Drawing for the job (mm, zero at the part's lowest x, y, z). A direction names the side the tool comes from. Give positions to 0.01 mm unless a question says otherwise; leave off trailing zeros. Write each loop counter-clockwise with the first axis right and the second up, starting at its lowest first coordinate (ties: lowest second). Pieces come first, ordered by that corner, then holes. Notation, with made-up numbers: M 20,59 L 79,59 A27 cw 79,97 Z; hole C 7.5,-16 d4. An arc over 180 degrees is marked long. Use CSV: the item, a comma, the result in double quotes. Start each with the question number.
1. Band-saw the part on B-B, the plane z = 3.75. List the corners of the cut face in (x, y).
2. Drop flat-ended pins along their axis: pin 1 Ø1.6 at (x, z) = (2.5, 2.5) entering from +Y; pin 2 Ø2 at (x, z) = (12, 2.5) entering from +Y; pin 3 Ø3.5 at (x, z) = (3.75, 11.25) entering from +Y. Give the stop position or say it passes through.
3. Band-saw the part on D-D, the plane y = 7.25. List the corners of the cut face in (x, z), then the cut area to 3 significant figures.
4. Mould opens along Z. For the marked faces 1, 2, 3 and 4 say: pulls with the +Z half, pulls with the -Z half, needs draft (parallel to the pull), parting line crosses it, or undercut.
5. Band-saw the part on C-C, the plane y = 3.5. Count the separate pieces of the cut face and the enclosed holes in it, then the cut area to 3 significant figures.
6. Drill centre lines: line 1 along Z through (x, y) = (3.75, 0.5); line 2 along X through (y, z) = (1.95, 3.75). Where is each one in solid material? Low to high. Write a range as from..to.
7. 3-axis set-ups, long thin cutter, end or side, ignore diameter. For the marked faces 5, 6 and 7: which of +Z, -Z, +X, -X, +Y, -Y reach the whole face in a straight line?
8. Band-saw the part on A-A, the plane x = 3.75. List the corners of the cut face in (y, z).
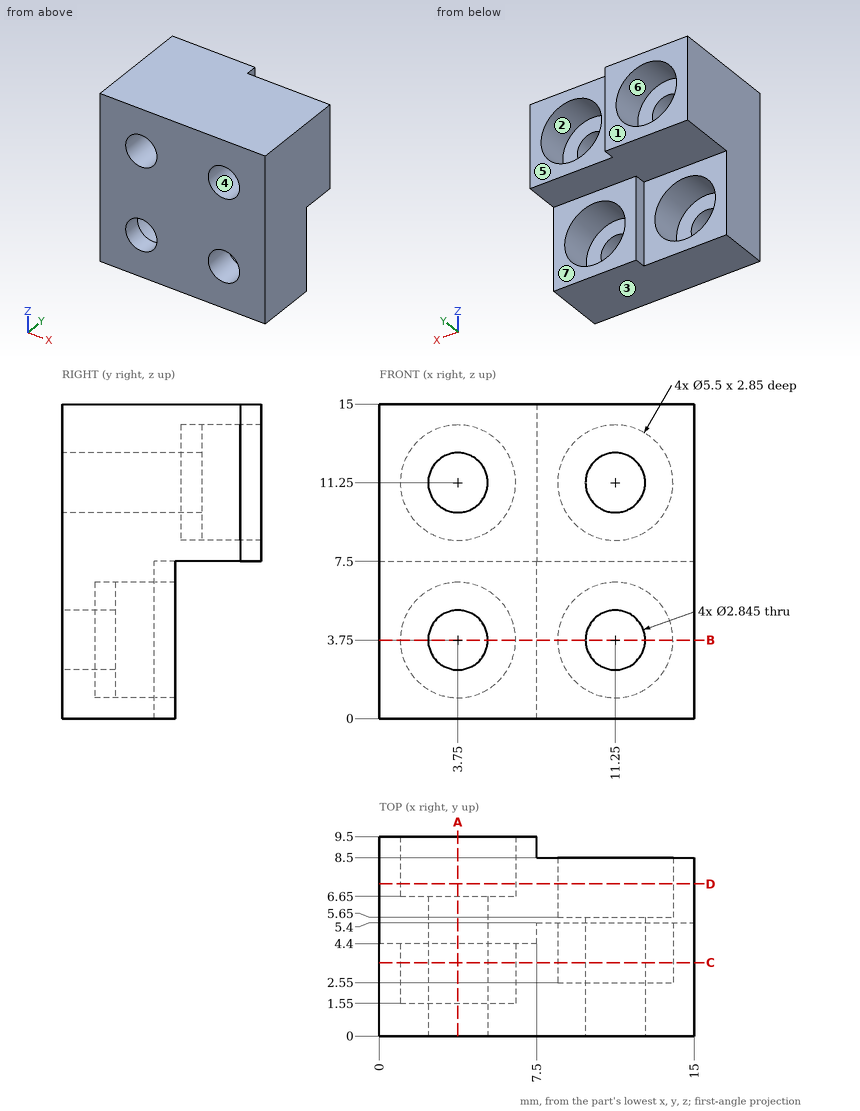
Output:
1,outline,"M 0,0 L 2.33,0 L 2.33,1.55 L 1,1.55 L 1,4.4 L 0,4.4 Z; M 5.17,0 L 9.83,0 L 9.83,2.55 L 8.5,2.55 L 8.5,5.4 L 7.5,5.4 L 7.5,4.4 L 6.5,4.4 L 6.5,1.55 L 5.17,1.55 Z; M 12.67,0 L 15,0 L 15,5.4 L 14,5.4 L 14,2.55 L 12.67,2.55 Z"
2,pin 1,"stops at y = 1.55"
2,pin 2,"stops at y = 2.55"
2,pin 3,"stops at y = 6.65"
3,outline,"M 0,7.5 L 15,7.5 L 15,15 L 0,15 Z; hole C 3.75,11.25 d5.5; hole C 11.25,11.25 d5.5"
3,area,"65.0 mm²"
4,face 1,"needs draft"
4,face 2,"undercut"
4,face 3,"pulls with the -Z half"
4,face 4,"undercut"
5,separate pieces,"1"
5,enclosed holes,"4"
5,area,"165 mm²"
6,line 1,"z = 0..2.33, 5.17..9.83, 12.67..15"
6,line 2,"x = 0..1, 6.5..9.83, 12.67..15"
7,face 5,"+Z, -Z, +X, +Y"
7,face 6,"+Y"
7,face 7,"-Z, +X, -X, +Y"
8,outline,"M 0,0 L 4.4,0 L 4.4,1 L 1.55,1 L 1.55,2.33 L 0,2.33 Z; M 0,5.17 L 1.55,5.17 L 1.55,6.5 L 4.4,6.5 L 4.4,7.5 L 9.5,7.5 L 9.5,8.5 L 6.65,8.5 L 6.65,9.83 L 0,9.83 Z; M 0,12.67 L 6.65,12.67 L 6.65,14 L 9.5,14 L 9.5,15 L 0,15 Z"
